Read the model definition and answer for the solid it produces. Units are mm, in the model's axes. A direction names the side the tool comes from. Coordinates: 2 decimals unless noted, no trailing zeros. Write each loop counter-clockwise with the first axis right and the second up, starting at its lowest first coordinate (ties: lowest second). Pieces come first, ordered by that corner, then holes. Notation, with made-up numbers: (13, 24) -> (50, 24) arc R19 ccw to (50, 29) -> close; hole circle Ø4 at (83, -36). An arc over 180 degrees is marked (long way). Write item = value, one per line. Start each with the question number.
1) Section D-D (z = -0.5) is taken. Determine the outline of the cut face in (x, y), plus the area to 3 significant figures.
2) A tool of negligible diameter and unlimited length cuts with its end or side. For faces 1 (the face through (18, 5, -7)), 2 (the face through (93.7, 0.2, 30)), 3 (the face through (48.134, -10.835, -6.527)), 4 (the face through (90, 0, 23)), 5 (the face through (55.197, -13.886, 18.661)), from which of +Z, -Z, +X, -X, +Y, -Y can it reach the whole face along a straight path? Write none if from no direction.
3) Section A-A (y = 0) is taken. Determine the outline of the cut face in (x, z), plus the area to 3 significant figures.
4) Section B-B (x = 0) is taken. Determine the outline of the cut face in (y, z), plus the area to 3 significant figures.
5) Flat-ended cylindrical pins translate along their axes: pin 1 Ø12 at (y, z) = (-7, 4) entering from -X; pin 2 Ø2 at (y, z) = (17.5, 12.5) entering from -X; pin 3 Ø5 at (y, z) = (11, 6.5) entering from +X. Find the tip coordinate at first contact, or state that the pin passes through.
6) Find the intervals of material crossed by line 1 along Y through (x, z) = (1, 5); line 2 along Z through (x, y) = (106, 2); line 3 along X through (y, z) = (0, -27), in increasing order. Write a range as from..to.
7) For a pull along X with two mould halves and no side action, classify faces 6 (the face through (46.877, 14.848, -0.147)), 7 (the face through (15.507, 15.606, 0.098)), 8 (the face through (19, 0, 7)) as released by +X, released by -X, zero draft, split by the parting line, or undercut.
8) Section C-C (x = 100) is taken. Determine the outline of the cut face in (y, z).
from build123d import *

# Parameters (mm, degrees)
SKETCH1_R               = 6
BOSS_EXTRUDE1_DEPTH     = 30
CUT_EXTRUDE1_DEPTH      = 61
SKETCH3_OUTSIDE_W       = 170.54
SKETCH3_OUTSIDE_H       = 93.54
CUT_EXTRUDE2_DEPTH      = 26
CUT_EXTRUDE2_DEPTH_BACK = 26
FILLET1_R               = 10


with BuildPart() as part:
    # Sketch1 → Boss-Extrude1 (new body, symmetric)
    with BuildSketch(Plane.XY):
        with BuildLine():
            Line((3.25, 24.787849846), (101.56, 11.898167926))
            ThreePointArc((101.56, 11.898167926), (112, 0), (101.56, -11.898167926))
            Line((101.56, -11.898167926), (3.25, -24.787849846))
            ThreePointArc((3.25, -24.787849846), (-25, 0), (3.25, 24.787849846))
        make_face()
        with Locations((100, 0)):
            Circle(SKETCH1_R, mode=Mode.SUBTRACT)
        with BuildLine():
            Line((8.691485355, 15.762553167), (12.02081528, 19.091883092))
            Line((12.02081528, 19.091883092), (19.091883092, 12.02081528))
            Line((19.091883092, 12.02081528), (15.762553167, 8.691485355))
            ThreePointArc((15.762553167, 8.691485355), (-12.727922061, -12.727922061), (8.691485355, 15.762553167))
        make_face(mode=Mode.SUBTRACT)
    extrude(amount=BOSS_EXTRUDE1_DEPTH, both=True)

    # Sketch2 → Cut-Extrude1 (cut, through all)
    with BuildSketch(Plane.XY.offset(30)):
        with BuildLine():
            Line((80.858, 6.543992359), (30.550654544, 13.139920354))
            ThreePointArc((30.550654544, 13.139920354), (26.131839925, 11.468082627), (25.077968327, 6.862616452))
            ThreePointArc((25.077968327, 6.862616452), (26, 0), (25.077968327, -6.862616452))
            ThreePointArc((25.077968327, -6.862616452), (26.131839925, -11.468082627), (30.550654544, -13.139920354))
            Line((30.550654544, -13.139920354), (80.858, -6.543992359))
            ThreePointArc((80.858, -6.543992359), (86.6, 0), (80.858, 6.543992359))
        make_face()
    extrude(amount=-CUT_EXTRUDE1_DEPTH, mode=Mode.SUBTRACT)

    # Sketch3 outside → Cut-Extrude2 (cut, two sides)
    with BuildSketch(Plane(origin=(0, 0, 0), x_dir=(1, 0, 0), z_dir=(0, 1, 0))) as cut_extrude2_sk:
        with Locations((43.5, 0)):
            Rectangle(SKETCH3_OUTSIDE_W, SKETCH3_OUTSIDE_H)
        Polygon((-25, 7), (35, 7), (74.837168574, 30), (112, 30), (112, 23), (76.712812921, 23), (36.875644347, 0), (76.712812921, -23), (112, -23), (112, -30), (74.837168574, -30), (35, -7), (-25, -7), align=None, mode=Mode.SUBTRACT)
    extrude(amount=CUT_EXTRUDE2_DEPTH, mode=Mode.SUBTRACT)
    extrude(cut_extrude2_sk.sketch, amount=-CUT_EXTRUDE2_DEPTH_BACK, mode=Mode.SUBTRACT)

    # Fillet1
    fillet1_edges = [part.edges().sort_by_distance(p)[0] for p in [
        (36.875644347, -16.344868893, 0),
        (36.875644347, 16.344868893, 0),
    ]]
    fillet(fillet1_edges, radius=FILLET1_R)


solid = part.part
Answer key:
q1.outline = (3.25, -24.79) -> (46.89, -19.07) -> (46.89, -11) -> (30.55, -13.14) arc R5 cw to (25.08, -6.86) arc R26 ccw to (25.08, 6.86) arc R5 cw to (30.55, 13.14) -> (46.89, 11) -> (46.89, 19.07) -> (3.25, 24.79) arc R25 ccw (long way) to start; hole (8.69, 15.76) arc R18 ccw (long way) to (15.76, 8.69) -> (19.09, 12.02) -> (12.02, 19.09) -> close
q1.area = 1,480 mm^2
q2.face_1 = -Z, -X, +Y, -Y
q2.face_2 = +Z, +X, -X, +Y, -Y
q2.face_3 = +Z, -Z
q2.face_4 = +X, +Y, -Y
q2.face_5 = +Z, -X, +Y, -Y
q3.outline = (-25, -7) -> (-18, -7) -> (-18, 7) -> (-25, 7) -> close; (18, -7) -> (26, -7) -> (26, 7) -> (18, 7) -> close; (86.6, -30) -> (94, -30) -> (94, -23) -> (86.6, -23) -> close; (86.6, 23) -> (94, 23) -> (94, 30) -> (86.6, 30) -> close; (106, -30) -> (112, -30) -> (112, -23) -> (106, -23) -> close; (106, 23) -> (112, 23) -> (112, 30) -> (106, 30) -> close
q3.area = 398 mm^2
q4.outline = (-25, -7) -> (-18, -7) -> (-18, 7) -> (-25, 7) -> close; (18, -7) -> (25, -7) -> (25, 7) -> (18, 7) -> close
q4.area = 196 mm^2
q5.pin_1 = -24.98
q5.pin_2 = 42.79
q5.pin_3 = 52.46
q6.line_1 = -24.98..-17.97, 17.97..24.98
q6.line_2 = -30..-23, 23..30
q6.line_3 = 86.6..94, 106..112
q7.face_6 = released by +X
q7.face_7 = undercut
q7.face_8 = zero draft
q8.outline = (-12.1, -30) -> (-6, -30) -> (-6, -23) -> (-12.1, -23) -> close; (-12.1, 23) -> (-6, 23) -> (-6, 30) -> (-12.1, 30) -> close; (6, -30) -> (12.1, -30) -> (12.1, -23) -> (6, -23) -> close; (6, 23) -> (12.1, 23) -> (12.1, 30) -> (6, 30) -> close
